Design review of the part built by this model. Coordinates are the model's own, in mm. A direction names the side the tool comes from. Give positions to 0.01 mm unless a question says otherwise; leave off trailing zeros. Loops run counter-clockwise (first coordinate to the right, second up) from the corner with the lowest first, then second, coordinate; pieces in that order, holes last.
from build123d import *

# Parameters (mm, degrees)
EXTRUDE_5_DEPTH        = 4.8
EXTRUDE_5_DEPTH_BACK   = 4
EXTRUDE_START          = -4
EXTRUDE_902_DEPTH      = 8.8
SKETCH_8_W             = 20
SKETCH_8_H             = 25
SKETCH_8_R             = 1.25
EXTRUDE_2674_DEPTH     = 2
CHAMFER_2_SIZE         = 1.5
CUT_EXTRUDE_2965_REACH = 28.131
SKETCH_9_R             = 2


with BuildPart() as part:
    # Эскиз1 → Выталкивающая часть (С ПАЗАМИ В ОБЕ СТОРОНЫ ВЫДАВИТЬ НА 5ММ) (new, two sides: drawn at the far end of the back side and taken through both)
    with BuildSketch(Plane.XY.offset(-EXTRUDE_5_DEPTH_BACK)):
        with BuildLine():
            ThreePointArc((-4.464770012, -5.712121212), (7.25, 0), (-4.464770012, 5.712121212))
            ThreePointArc((-4.464770012, 5.712121212), (-5.868479146, 5.884169654), (-5.696430705, 7.287878788))
            ThreePointArc((-5.696430705, 7.287878788), (9.25, 0), (-5.696430705, -7.287878788))
            ThreePointArc((-5.696430705, -7.287878788), (-5.868479146, -5.884169654), (-4.464770012, -5.712121212))
        make_face()
    extrude(amount=EXTRUDE_5_DEPTH + EXTRUDE_5_DEPTH_BACK)

    # Эскиз2 → Extrude 902 (add)
    with BuildSketch(Plane.XY.offset(EXTRUDE_START)):
        with BuildLine():
            Line((12.5, 3.75), (12.5, -3.75))
            ThreePointArc((12.5, -3.75), (9.598284348, -4.027802018), (7.246080423, -5.749505936))
            ThreePointArc((7.246080423, -5.749505936), (9.25, 0), (7.246080423, 5.749505936))
            ThreePointArc((7.246080423, 5.749505936), (9.598284348, 4.027802018), (12.5, 3.75))
        make_face()
    extrude(amount=EXTRUDE_902_DEPTH)

    # Эскиз8 → Extrude 2674 (add)
    with BuildSketch(Plane(origin=(12.5, 0, 0), x_dir=(0, 0, -1), z_dir=(1, 0, 0))):
        with Locations((-0.15, 0)):
            Rectangle(SKETCH_8_W, SKETCH_8_H)
        with Locations((-7.65, 10)):
            Circle(SKETCH_8_R, mode=Mode.SUBTRACT)
        with Locations((-7.65, -10)):
            Circle(SKETCH_8_R, mode=Mode.SUBTRACT)
        with Locations((7.35, -10)):
            Circle(SKETCH_8_R, mode=Mode.SUBTRACT)
        with Locations((7.35, 10)):
            Circle(SKETCH_8_R, mode=Mode.SUBTRACT)
    extrude(amount=EXTRUDE_2674_DEPTH)

    # Фаска2
    # the kernel refuses this chamfer: 1.5 mm, written as the material it takes off along each edge
    with BuildSketch(Plane(origin=(14.5, -10, -7.35), x_dir=(0, 0, -1), z_dir=(0, -1, 0))) as chamfer_2_piece_1:
        Polygon((1.25 + CHAMFER_2_SIZE, 0), (1.25, -CHAMFER_2_SIZE), (1.25, 0), align=None)
    revolve(axis=Axis((14.5, -10, -7.35), (1, 0, 0)), mode=Mode.SUBTRACT)
    with BuildSketch(Plane(origin=(14.5, 10, 7.65), x_dir=(0, 0, -1), z_dir=(0, -1, 0))) as chamfer_2_piece_2:
        Polygon((1.25 + CHAMFER_2_SIZE, 0), (1.25, -CHAMFER_2_SIZE), (1.25, 0), align=None)
    revolve(axis=Axis((14.5, 10, 7.65), (1, 0, 0)), mode=Mode.SUBTRACT)
    with BuildSketch(Plane(origin=(14.5, -10, 7.65), x_dir=(0, 0, -1), z_dir=(0, -1, 0))) as chamfer_2_piece_3:
        Polygon((1.25 + CHAMFER_2_SIZE, 0), (1.25, -CHAMFER_2_SIZE), (1.25, 0), align=None)
    revolve(axis=Axis((14.5, -10, 7.65), (1, 0, 0)), mode=Mode.SUBTRACT)
    with BuildSketch(Plane(origin=(14.5, 10, -7.35), x_dir=(0, 0, -1), z_dir=(0, -1, 0))) as chamfer_2_piece_4:
        Polygon((1.25 + CHAMFER_2_SIZE, 0), (1.25, -CHAMFER_2_SIZE), (1.25, 0), align=None)
    revolve(axis=Axis((14.5, 10, -7.35), (1, 0, 0)), mode=Mode.SUBTRACT)

    # Эскиз9 → Cut-Extrude 2965 (cut, up to next)
    with BuildSketch(Plane(origin=(14.5, 0, 0), x_dir=(0, 0, -1), z_dir=(1, 0, 0)), mode=Mode.PRIVATE) as cut_extrude_2965_sk1:
        with Locations((3.5, 0)):
            Circle(SKETCH_9_R)
    cut_extrude_2965_tool1 = extrude(cut_extrude_2965_sk1.sketch, amount=-CUT_EXTRUDE_2965_REACH, mode=Mode.PRIVATE) & part.part
    add(cut_extrude_2965_tool1.solids().sort_by_distance((14.5, 0, -3.5))[0], mode=Mode.SUBTRACT)


solid = part.part
Q1. Take a section at A-A (y = 0). Give the boundary of the cut face in (x, z).
Results:
outline: (7.25, -1.5) - (14.5, -1.5) - (14.5, 10.15) - (12.5, 10.15) - (12.5, 4.8) - (7.25, 4.8) - close; (12.5, -9.85) - (14.5, -9.85) - (14.5, -5.5) - (12.5, -5.5) - close
Q2. Wall thickness on line 1 (Y direction, x = 12.85, z = 7.65); line 2 (X direction, y = 0, z = 1.25); line 3 (Y direction, x = 0, z = -0.5): over which ranges is each line inside the solid? List them lowest first.
Results:
line 1: y = -12.5 to -11.25, -8.75 to 8.75, 11.25 to 12.5
line 2: x = 7.25 to 14.5
line 3: y = -9.25 to -7.25, 7.25 to 9.25
Q3. Insertion check: pin 1 (1.5 mm diameter, centred on y = 1.5, z = -2.5, fed in from +X); pin 2 (3 mm diameter, centred on x = 10.5, z = 4, fed in from -Y); pin 3 (8 mm diameter, centred on x = -3.5, z = 4, fed in from +Y); pin 4 (3 mm diameter, centred on y = -10, z = -7.35, fed in from -X). Each pin has a flat end and moves straight along its axis. Give the tip position at first contact, or say it passes through.
Results:
pin 1: stops at x = 14.5
pin 2: stops at y = -4.3
pin 3: stops at y = 9.25
pin 4: stops at x = 12.5
Q4. Tool access review of faces 4 (the face through (12.75, 11.24, 7.81)), 5 (the face through (4, -7, -4)): name each direction out of +Z, -Z, +X, -X, +Y, -Y from which nothing blocks a thin tool from reaching the whole face with its end or side.
Results:
face 4: +X, -X
face 5: -Z, -X, +Y, -Y
Q5. Take a section at B-B (y = -10). Give the boundary of the cut face in (x, z).
Results:
outline: (12.5, -9.85) - (14.25, -9.85) - (13, -8.6) - (12.5, -8.6) - close; (12.5, -6.1) - (13, -6.1) - (14.5, -4.6) - (14.5, 4.9) - (13, 6.4) - (12.5, 6.4) - close; (12.5, 8.9) - (13, 8.9) - (14.25, 10.15) - (12.5, 10.15) - close
Q6. Draft analysis for pull direction X (two halves, no side actions). For faces 1 (the face through (12.5, 3, -4.2)), 2 (the face through (14.5, -12.1, -9.5)), 3 (the face through (7.4, -0.6, 4.8)), state which applies: pulls with the +X half, pulls with the -X half, needs draft (parallel to the pull), parting line crosses it, or undercut.
Results:
face 1: undercut
face 2: pulls with the +X half
face 3: needs draft
Q7. Take a section at C-C (z = 7.65). Give the boundary of the cut face in (x, y), plus the area to 3 significant figures.
Results:
outline: (12.5, -12.5) - (14.25, -12.5) - (13, -11.25) - (12.5, -11.25) - close; (12.5, -8.75) - (13, -8.75) - (14.5, -7.25) - (14.5, 7.25) - (13, 8.75) - (12.5, 8.75) - close; (12.5, 11.25) - (13, 11.25) - (14.25, 12.5) - (12.5, 12.5) - close
area: 35.6 mm2
Q8. Take a section at D-D (x = 0). Give the boundary of the cut face in (y, z).
Results:
outline: (-9.25, -4) - (-7.25, -4) - (-7.25, 4.8) - (-9.25, 4.8) - close; (7.25, -4) - (9.25, -4) - (9.25, 4.8) - (7.25, 4.8) - close
